Autodesk Inventor part; units mm, degrees
ref_plane "YZ Plane" through (0, 0, 0) normal (1, 0, 0) x (0, 1, 0)
ref_plane "XZ Plane" through (0, 0, 0) normal (0, 1, 0) x (-1, 0, 0)
ref_plane "XY Plane" through (0, 0, 0) normal (0, 0, 1) x (1, 0, 0)
sketch "スケッチ1" plane through (0, 0, 0) normal (0, 0, 1) x (1, 0, 0)
  circle A0 centre (0, 0) radius 14
  dimension "d0" = 28
extrude "押し出し1" add sketch "スケッチ1" along normal blind 19
sketch "スケッチ2" plane through (0, 0, 19) normal (0, 0, 1) x (1, 0, 0)
  circle A0 centre (0, 0) radius 14
  arc A1 (-17.5, 3.5) -> (-17.5, -3.5) centre (-17.5, 0) ccw
  arc A2 (17.5, -3.5) -> (17.5, 3.5) centre (17.5, 0) ccw
  line L0 (-17.5, 3.5) -> (-13.5554, 3.5)
  line L1 (-17.5, -3.5) -> (-13.5554, -3.5)
  line L2 (13.5554, 3.5) -> (17.5, 3.5)
  line L3 (13.5554, -3.5) -> (17.5, -3.5)
  circle A3 centre (-17.5, 0) radius 2
  circle A4 centre (17.5, 0) radius 2
  dimension "d5" = 7
  dimension "d6" = 7
  dimension "d7" = 4
  dimension "d8" = 4
extrude "押し出し2" add sketch "スケッチ2" against normal blind 0.9 contours A0 L2 A2 L3 | A0 L1 A1 L0
sketch "スケッチ3" plane through (0, 0, 19) normal (0, 0, 1) x (1, 0, 0)
  line L0 (-7.25, -14) -> (-7.25, -18)
  line L1 (-7.25, -18) -> (7.25, -18)
  line L2 (7.25, -18) -> (7.25, -14)
  line L3 (-7.25, -14) -> (-7.25, -12.0918)
  line L4 (7.25, -14) -> (7.25, -12.0918)
  circle A0 centre (-17.5, 0) radius 2
  circle A1 centre (17.5, 0) radius 2
  arc A2 (13.5554, 3.5) -> (-13.5554, 3.5) centre (0, 0) ccw
  line L5 (-13.5554, 3.5) -> (-17.5, 3.5)
  arc A3 (-17.5, 3.5) -> (-17.5, -3.5) centre (-17.5, 0) ccw
  line L6 (-17.5, -3.5) -> (-13.5554, -3.5)
  arc A4 (-13.5554, -3.5) -> (13.5554, -3.5) centre (0, 0) ccw
  line L7 (13.5554, -3.5) -> (17.5, -3.5)
  arc A5 (17.5, -3.5) -> (17.5, 3.5) centre (17.5, 0) ccw
  line L8 (17.5, 3.5) -> (13.5554, 3.5)
  line L9 (7.25, -12.0918) -> (-7.25, -12.0918)
  line L10 (-7.25, -12.0918) -> (-7.25, -18)
  line L11 (-7.25, -18) -> (7.25, -18)
  line L12 (7.25, -18) -> (7.25, -12.0918)
extrude "押し出し3" add sketch "スケッチ3" against normal blind 16.5 contours L3 L9 A4 L4 L2 L1 L0 | L9 A4
sketch "スケッチ4" plane through (0, 0, 19) normal (0, 0, 1) x (1, 0, 0)
  arc A0 (7.056, -12.0918) -> (13.5554, -3.5) centre (0, 0) ccw
  line L0 (13.5554, -3.5) -> (17.5, -3.5)
  arc A1 (17.5, -3.5) -> (17.5, 3.5) centre (17.5, 0) ccw
  line L1 (17.5, 3.5) -> (13.5554, 3.5)
  arc A2 (13.5554, 3.5) -> (-13.5554, 3.5) centre (0, 0) ccw
  line L2 (-13.5554, 3.5) -> (-17.5, 3.5)
  arc A3 (-17.5, 3.5) -> (-17.5, -3.5) centre (-17.5, 0) ccw
  line L3 (-17.5, -3.5) -> (-13.5554, -3.5)
  arc A4 (-13.5554, -3.5) -> (-7.056, -12.0918) centre (0, 0) ccw
  line L4 (-7.25, -12.0918) -> (-7.056, -12.0918)
  line L5 (-7.25, -18) -> (-7.25, -12.0918)
  line L6 (7.25, -18) -> (-7.25, -18)
  line L7 (7.25, -12.0918) -> (7.25, -18)
  line L8 (7.056, -12.0918) -> (7.25, -12.0918)
  circle A5 centre (-17.5, 0) radius 2
  circle A6 centre (17.5, 0) radius 2
  circle A7 centre (0, 7.25) radius 4.75
  dimension "d15" = 9.5
extrude "押し出し4" add sketch "スケッチ4" along normal blind 1.7 contours A7
sketch "スケッチ5" plane through (0, 7.25, 20.7) normal (0, 0, 1) x (1, 0, 0)
  circle A0 centre (0, 0) radius 2.5
  point P0 (0, -7.25)
  dimension "d18" = 5
extrude "押し出し5" add sketch "スケッチ5" along normal blind 8
sketch "スケッチ6" plane through (0, 7.25, 28.7) normal (0, 0, 1) x (1, 0, 0)
  circle A0 centre (0, 0) radius 2.5
  line L0 (2, 1.5) -> (-2, 1.5)
  line L1 (-2, -1.5) -> (2, -1.5)
  circle A1 centre (0, 0) radius 2.5
  point P0 (0, -7.25)
  dimension "d23" = 5
extrude "押し出し6" cut sketch "スケッチ6" against normal blind 6 contours L0 A0 | A0 L1
sketch "スケッチ7" plane through (-7.25, -18, 19) normal (0, -1, 0) x (1, 0, 0)
  line L0 (3.75, -1.5) -> (10.75, -1.5)
  line L1 (10.75, -1.5) -> (10.75, -3)
  line L2 (10.75, -3) -> (3.75, -3)
  line L3 (3.75, -3) -> (3.75, -1.5)
  point P0 (7.25, -19)
  dimension "d26" = 7
  dimension "d27" = 1.5
extrude "押し出し7" cut sketch "スケッチ7" against normal blind 5
sketch "スケッチ8" plane through (0, 0, 19) normal (0, 0, 1) x (1, 0, 0)
  circle A0 centre (0, 7.25) radius 4.75
  arc A1 (7.056, -12.0918) -> (13.5554, -3.5) centre (0, 0) ccw
  line L0 (13.5554, -3.5) -> (17.5, -3.5)
  arc A2 (17.5, -3.5) -> (17.5, 3.5) centre (17.5, 0) ccw
  line L1 (17.5, 3.5) -> (13.5554, 3.5)
  arc A3 (13.5554, 3.5) -> (-13.5554, 3.5) centre (0, 0) ccw
  line L2 (-13.5554, 3.5) -> (-17.5, 3.5)
  arc A4 (-17.5, 3.5) -> (-17.5, -3.5) centre (-17.5, 0) ccw
  line L3 (-17.5, -3.5) -> (-13.5554, -3.5)
  arc A5 (-13.5554, -3.5) -> (-7.056, -12.0918) centre (0, 0) ccw
  line L4 (-7.25, -12.0918) -> (-7.056, -12.0918)
  line L5 (-7.25, -18) -> (-7.25, -12.0918)
  line L6 (7.25, -18) -> (-7.25, -18)
  line L7 (7.25, -12.0918) -> (7.25, -18)
  line L8 (7.056, -12.0918) -> (7.25, -12.0918)
  circle A6 centre (-17.5, 0) radius 2
  circle A7 centre (17.5, 0) radius 2
sketch "スケッチ9" plane through (0, 0, 19) normal (0, 0, 1) x (1, 0, 0)
  circle A0 centre (-17.5, 0) radius 2
  circle A1 centre (-17.5, 0) radius 2
  circle A2 centre (0, 7.25) radius 4.75
  circle A3 centre (0, 7.25) radius 4.75
  circle A4 centre (17.5, 0) radius 2
  circle A5 centre (17.5, 0) radius 2
  point P0 (0, 0)
properties part number "28BYJ-48" material "鋼"
Could you check a few things on this model? Use its own coordinates, in mm. A direction names the side the tool comes from. Give positions to 0.01 mm unless a question says otherwise; leave off trailing zeros. Order: outer loops, then holes, each group sorted by start corner. A loop starts at its lowest first (then second) coordinate and runs counter-clockwise, first axis right, second up. Notation, with made-up numbers: (62.25, 74) -> (66.25, 74) arc R28 ccw to (66.25, 102) -> close; hole circle Ø4 at (-20.5, 24). An arc over 180 degrees is marked (long way). Answer in a Markdown table with one row per item. Add a question column.
Item 1: Imagine slicing it at D-D (y = 1). List the corners of the cut face in (x, z) for me.
Item 2: For faces 1 (the cylindrical face through (4.53, 5.82, 19.84)), 2 (the cylindrical face through (-21, 0.1, 18.6)), 3 (the flat face through (3.5, -16, 17)), 4 (the flat face through (7.25, -15, 11)), 5 (the cylindrical face through (15.9, -1.2, 18.6)), which set-ups out of +Z, -Z, +X, -X, +Y, -Y let a thin tool reach every point of the face, with its end or its side?
Item 3: Imagine slicing it at B-B (z = 12.25). List the corners of the cut face in (x, y) for me.
Item 4: Imagine slicing it at A-A (x = 0). List the corners of the cut face in (y, z) for me, and give its area (3 significant figures).
Item 5: I'm going to push flat-ended pins straight in: P1, Ø8, axis at x = -16.5, y = -12, coming from the -Z side; P2, Ø1, axis at y = -9, z = 12.5, coming from the +X side; P3, Ø5, axis at x = 9, z = 9, coming from the +Y side; P4, Ø3.5, axis at x = -18.5, y = 0, coming from the -Z side. Where does each tip first touch, or does it pass through?
Item 6: We'd pull the mould along Y, two halves only. Please class faces 6 (the cylindrical face through (-19.1, -1.2, 18.6)), 7 (the flat face through (0, 9, 22.7)), 8 (the flat face through (0, 8.75, 26)), 9 (the flat face through (0, 5.75, 26)): pulls with the +Y half, pulls with the -Y half, needs draft (parallel to the pull), parting line crosses it, or undercut.
Item 7: Please list where these lines run through material, in increasing order: probe 1 along Z at (x, y) = (-2.5, -15); probe 2 along Y at (x, z) = (-17.5, 18.7); probe 3 along X at (y, z) = (7, 27.5).
Item 8: Imagine slicing it at C-C (y = 7.25). List the corners of the cut face in (x, z) for me, and give its area (3 significant figures).
Result:
| question | item | result |
|---|---|---|
| 1 | outline | (-20.85, 18.1) -> (-19.23, 18.1) -> (-19.23, 19) -> (-20.85, 19) -> close; (-15.77, 18.1) -> (-13.96, 18.1) -> (-13.96, 0) -> (13.96, 0) -> (13.96, 18.1) -> (15.77, 18.1) -> (15.77, 19) -> (-15.77, 19) -> close; (19.23, 18.1) -> (20.85, 18.1) -> (20.85, 19) -> (19.23, 19) -> close |
| 2 | face 1 | +Z |
| 2 | face 2 | +Z, -Z, -X |
| 2 | face 3 | -Y |
| 2 | face 4 | +Z, -Z, +X, -Y |
| 2 | face 5 | +Z, -Z |
| 3 | outline | (-7.25, -18) -> (7.25, -18) -> (7.25, -12.09) -> (7.06, -12.09) arc R14 ccw (long way) to (-7.06, -12.09) -> (-7.25, -12.09) -> close |
| 4 | outline | (-18, 2.5) -> (-14, 2.5) -> (-14, 0) -> (14, 0) -> (14, 19) -> (12, 19) -> (12, 20.7) -> (9.75, 20.7) -> (9.75, 22.7) -> (8.75, 22.7) -> (8.75, 28.7) -> (5.75, 28.7) -> (5.75, 22.7) -> (4.75, 22.7) -> (4.75, 20.7) -> (2.5, 20.7) -> (2.5, 19) -> (-18, 19) -> (-18, 17.5) -> (-13, 17.5) -> (-13, 16) -> (-18, 16) -> close |
| 4 | area | 635 mm2 |
| 5 | P1 | through |
| 5 | P2 | x = 11.12 |
| 5 | P3 | y = 12.4 |
| 5 | P4 | z = 18.1 |
| 6 | face 6 | undercut |
| 6 | face 7 | needs draft |
| 6 | face 8 | pulls with the +Y half |
| 6 | face 9 | pulls with the -Y half |
| 7 | probe 1 | 2.5 to 16, 17.5 to 19 |
| 7 | probe 2 | -3.5 to -2, 2 to 3.5 |
| 7 | probe 3 | -2.49 to 2.49 |
| 8 | outline | (-11.98, 0) -> (11.98, 0) -> (11.98, 19) -> (4.75, 19) -> (4.75, 20.7) -> (2.5, 20.7) -> (2.5, 28.7) -> (-2.5, 28.7) -> (-2.5, 20.7) -> (-4.75, 20.7) -> (-4.75, 19) -> (-11.98, 19) -> close |
| 8 | area | 511 mm2 |
